```python
from build123d import *


with BuildPart() as f1:
    # F0 (on Front) → F1 (revolve)
    with BuildSketch(Plane.XZ):
        Polygon((0, 5.806352), (0, 20.549649), (-31.5, 20.549649), (-31.5, 100), (-34.5, 100), (-34.5, 15.603564), (-23.352671, 15.603564), (-23.352671, 5.806352), align=None)
        Polygon((31.5, 20.549649), (0, 20.549649), (0, 5.806352), (23.352671, 5.806352), (23.352671, 15.603564), (34.5, 15.603564), (34.5, 100), (31.5, 100), align=None)
    revolve(axis=Axis((6.947005, 0, 0), (1, 0, 0)))


solid = f1.part
```
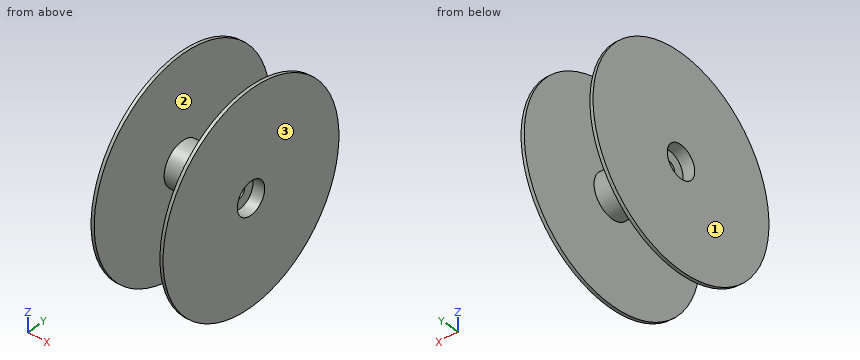
The listing builds one solid part. Answer for the finished solid, in the listing's coordinates (mm). Face numbers are marked on the shaded views. Give positions to 0.01 mm unless a question says otherwise; leave off trailing zeros. Order: outer loops, then holes, each group sorted by start corner. A loop starts at its lowest first (then second) coordinate and runs counter-clockwise, first axis right, second up. Notation, with made-up numbers: (20, 23.25) -> (73, 23.25) arc R30 cw to (73, 57.25) -> close; hole circle Ø4 at (63, 84). An arc over 180 degrees is marked (long way). Answer as a JSON object with one key per item and string values. Group by question number.
Item 1: Consider L1, parallel to Z at x = -9, y = 0; L2, parallel to Z at x = 26.25, y = 0; L3, parallel to X at y = -27, z = -92. Determine where each line is inside the solid, lowest interval first. Write a range as from..to.
Item 2: Determine the mould class of the marked faces 1, 2 and 3 for opening direction X: pulls with the +X half, pulls with the -X half, needs draft (parallel to the pull), parting line crosses it, or undercut.
Item 3: The part is cut by section A-A on y = 0. Write down the section's boundary in (x, z).
Item 4: The part is cut by section C-C on x = 28. Write down the section's boundary in (y, z).
Item 5: The part is cut by section D-D on y = 34. Write down the section's boundary in (x, z).
Item 6: Flat-ended cylindrical pins translate along their axes: pin 1 (9.5 mm diameter, centred on y = 6, z = -7.5, fed in from +X); pin 2 (10.5 mm diameter, centred on y = 0, z = 0, fed in from -X); pin 3 (12 mm diameter, centred on x = 21, z = -22.5, fed in from +Y); pin 4 (15.5 mm diameter, centred on y = 1.5, z = -2, fed in from -X). Find the tip coordinate at first contact, or state that the pin passes through.
Result set:
{
 "1": {"L1": "-20.55..-5.81, 5.81..20.55", "L2": "-20.55..-15.6, 15.6..20.55", "L3": "-34.5..-31.5, 31.5..34.5"},
 "2": {"face 1": "pulls with the -X half", "face 2": "undercut", "face 3": "pulls with the +X half"},
 "3": {"outline": "(-34.5, -100) -> (-31.5, -100) -> (-31.5, -20.55) -> (31.5, -20.55) -> (31.5, -100) -> (34.5, -100) -> (34.5, -15.6) -> (23.35, -15.6) -> (23.35, -5.81) -> (-23.35, -5.81) -> (-23.35, -15.6) -> (-34.5, -15.6) -> close; (-34.5, 15.6) -> (-23.35, 15.6) -> (-23.35, 5.81) -> (23.35, 5.81) -> (23.35, 15.6) -> (34.5, 15.6) -> (34.5, 100) -> (31.5, 100) -> (31.5, 20.55) -> (-31.5, 20.55) -> (-31.5, 100) -> (-34.5, 100) -> close"},
 "4": {"outline": "circle Ø41.1 at (0, 0); hole circle Ø31.21 at (0, 0)"},
 "5": {"outline": "(-34.5, -94.04) -> (-31.5, -94.04) -> (-31.5, 94.04) -> (-34.5, 94.04) -> close; (31.5, -94.04) -> (34.5, -94.04) -> (34.5, 94.04) -> (31.5, 94.04) -> close"},
 "6": {"pin 1": "x = 23.35", "pin 2": "through", "pin 3": "y = 12.25", "pin 4": "x = -23.35"}
}
